Read the model definition and answer for the solid it produces. Units are mm, in the model's axes. A direction names the side the tool comes from. Give positions to 0.01 mm unless a question says otherwise; leave off trailing zeros. Loops run counter-clockwise (first coordinate to the right, second up) from the corner with the lowest first, then second, coordinate; pieces in that order, holes last. Notation, with made-up numbers: (9, 59) -> (37, 59) arc R15 cw to (37, 84) -> close; hole circle Ø5 at (-33.75, 35). An arc over 180 degrees is marked (long way). Answer as CSV lines item,"result". Start each with the question number.
```python
from build123d import *

# Parameters (mm, degrees)
BOSS_EXTRUDE1_DEPTH     = 177.8
F_1_4_20_TAPPED_HOLE1_D = 5.1054


with BuildPart() as part:
    # Sketch2 → Boss-Extrude1 (new, symmetric)
    with BuildSketch(Plane.XY):
        Polygon((-16.66875, 12.7), (-19.05, 12.7), (-19.05, 0), (19.05, 0), (19.05, 12.7), (16.66875, 12.7), (16.66875, 2.38125), (-16.66875, 2.38125), align=None)
    extrude(amount=BOSS_EXTRUDE1_DEPTH, both=True)

    # 1/4-20 Tapped Hole1 (through all)
    with Locations(Plane(origin=(0, 2.38125, 0), x_dir=(1, 0, 0), z_dir=(0, 1, 0))):
        with Locations((0, -165.1)):
            f_1_4_20_tapped_hole1 = Hole(F_1_4_20_TAPPED_HOLE1_D / 2)

    # Mirror1: 1/4-20 Tapped Hole1 across plane
    add(f_1_4_20_tapped_hole1.mirror(Plane.XY), mode=Mode.SUBTRACT)


solid = part.part
```
(1) Find the intervals of material crossed by line 1 along Z through (x, y) = (0, 1.75); line 2 along X through (y, z) = (1.6, -165.1); line 3 along X through (y, z) = (11.75, 109), in increasing order. Write a range as from..to.
(2) The mould has two halves that part along X. Classify faces 1 (the face through (0, 2.381, 2)), 2 (the face through (0, 2, -177.8)), 3 (the face through (19.05, 6, 2)), 4 (the face through (16.669, 8, 2)): pulls with the +X half, pulls with the -X half, needs draft (parallel to the pull), parting line crosses it, or undercut.
(3) Find section A-A on y = 8.25. Write down the section's boundary in (x, z).
(4) Find section B-B on z = 49. Write down the section's boundary in (x, y), then the cut area to 3 significant figures.
(5) Find section C-C on x = 11.5. Write down the section's boundary in (y, z).
(6) A tool of negligible diameter and unlimited length cuts with its end or side. For faces 5 (the face through (-16.669, 7, 2)), 6 (the face through (0, 0, 2)), from which of +Z, -Z, +X, -X, +Y, -Y can it reach the whole face along a straight path? Write none if from no direction.
(7) Each of these flat-tipped pins is pushed along its axis until it touches: P1, Ø4, axis at x = 3, z = -114.5, coming from the +Y side; P2, Ø4, axis at x = -14, y = 6, coming from the +Z side. Where does it stop, or does it pass through?
Answer block:
1,line 1,"z = -177.8..-167.65, -162.55..162.55, 167.65..177.8"
1,line 2,"x = -19.05..-2.55, 2.55..19.05"
1,line 3,"x = -19.05..-16.67, 16.67..19.05"
2,face 1,"undercut"
2,face 2,"needs draft"
2,face 3,"pulls with the +X half"
2,face 4,"undercut"
3,outline,"(-19.05, -177.8) -> (-16.67, -177.8) -> (-16.67, 177.8) -> (-19.05, 177.8) -> close; (16.67, -177.8) -> (19.05, -177.8) -> (19.05, 177.8) -> (16.67, 177.8) -> close"
4,outline,"(-19.05, 0) -> (19.05, 0) -> (19.05, 12.7) -> (16.67, 12.7) -> (16.67, 2.38) -> (-16.67, 2.38) -> (-16.67, 12.7) -> (-19.05, 12.7) -> close"
4,area,"140 mm2"
5,outline,"(0, -177.8) -> (2.38, -177.8) -> (2.38, 177.8) -> (0, 177.8) -> close"
6,face 5,"+Z, -Z, +Y"
6,face 6,"+Z, -Z, +X, -X, -Y"
7,P1,"stops at y = 2.38"
7,P2,"passes through"
